For this review, take the finished solid that the model builds, in its own axes (mm). Face numbers are marked on the shaded views. A direction names the side the tool comes from. Coordinates: 2 decimals unless noted, no trailing zeros. Loops run counter-clockwise (first coordinate to the right, second up) from the corner with the lowest first, then second, coordinate; pieces in that order, holes last. Notation, with made-up numbers: M -14.5,31 L 26.5,31 A29 ccw 26.5,59 Z; hole C 11,21 d7. An arc over 180 degrees is marked long. Answer as a JSON object with one key per item and string values. Group by question number.
Item 1: Tool access review of the marked faces 1 and 2: name each direction out of +Z, -Z, +X, -X, +Y, -Y from which nothing blocks a thin tool from reaching the whole face with its end or side.
Item 2: Add section C-C (y = 19). State the section outline as (x, z) points.
Item 3: Add section A-A (y = 7). State the section outline as (x, z) points, then the cut area to 3 significant figures.
Item 4: Add section D-D (x = -3.75). State the section outline as (y, z) points, then the cut area to 3 significant figures.
Item 5: Add section B-B (z = 3). State the section outline as (x, y) points, then the cut area to 3 significant figures.
Item 6: Mouldability with a two-part tool opening along Z and no side actions: class the marked faces 3, 4, 5 and 6 as +Z half, -Z half, draft (parallel to the pull), parting line (faces both ways), or undercut.
Item 7: Wall thickness on L1, parallel to X at y = 1.75, z = 0; L2, parallel to Z at x = 6.5, y = 21.5; L3, parallel to X at y = 0.9, z = 3: over which ranges is each line inside the solid? List them lowest first. Write a range as from..to.
Item 8: Insertion check: pin 1 (5 mm diameter, centred on x = 1.5, z = 0, fed in from +Y); pin 2 (2 mm diameter, centred on y = 20.5, z = -12.5, fed in from +X); pin 3 (2.5 mm diameter, centred on x = 0, z = 3, fed in from +Y); pin 4 (3.5 mm diameter, centred on y = 1.5, z = 1.5, fed in from +X). Each pin has a flat end and moves straight along its axis. Give the tip position at first contact, or say it passes through.
from build123d import *

# Parameters (mm, degrees)
SKETCH_1_W          = 17
SKETCH_1_H          = 23.4
SKETCH_1_R          = 1.6
EXTRUDE_1_DEPTH     = 3
EXTRUDE_3_DEPTH     = 45
SKETCH_3_R          = 1.1
SKETCH_3_R_2        = 5
CUT_EXTRUDE_1_DEPTH = 45
FILLET_1_R          = 2
SKETCH_4_W          = 10
SKETCH_4_H          = 11.187827488
CUT_EXTRUDE_2_DEPTH = 29


with BuildPart() as part:
    # 草图1 → 凸台-拉伸1 (new body)
    with BuildSketch(Plane(origin=(0, 0, 0), x_dir=(1, 0, 0), z_dir=(0, 1, 0))):
        Rectangle(SKETCH_1_W, SKETCH_1_H)
        with Locations(Location((0, 3, 0), (0, 0, 270))):
            Circle(SKETCH_1_R, mode=Mode.SUBTRACT)
        with Locations(Location((-3, 0, 0), (0, 0, 270))):
            Circle(SKETCH_1_R, mode=Mode.SUBTRACT)
        with Locations(Location((0, -3, 0), (0, 0, 90))):
            Circle(SKETCH_1_R, mode=Mode.SUBTRACT)
        with Locations(Location((3, 0, 0), (0, 0, 90))):
            Circle(SKETCH_1_R, mode=Mode.SUBTRACT)
    extrude(amount=EXTRUDE_1_DEPTH)

    # 草图2 → 凸台-拉伸3 (add)
    with BuildSketch(Plane.XZ):
        Polygon((-8.5, 11.7), (-8.5, 13.7), (8.584010661, 13.7), (8.5, 11.7), align=None)
        Polygon((8.584010661, -13.7), (8.5, -11.7), (-8.5, -11.7), (-8.5, -13.7), align=None)
    extrude(amount=-EXTRUDE_3_DEPTH)

    # 草图3 → 切除-拉伸1 (cut)
    with BuildSketch(Plane.XY.offset(13.7)):
        with Locations((-5.707994669, 41)):
            Circle(SKETCH_3_R)
        with Locations((5.792005331, 41)):
            Circle(SKETCH_3_R)
        with Locations((0.042005331, 14)):
            Circle(SKETCH_3_R_2)
        with Locations((-5.707994669, 7)):
            Circle(SKETCH_3_R)
        with Locations((5.792005331, 7)):
            Circle(SKETCH_3_R)
    extrude(amount=-CUT_EXTRUDE_1_DEPTH, mode=Mode.SUBTRACT)

    # 圆角1
    fillet_1_edges = [part.edges().sort_by_distance(p)[0] for p in [
        (-8.5, 45, 12.7),
        (8.542005331, 45, 12.7),
        (-8.5, 45, -12.7),
        (8.542005331, 45, -12.7),
    ]]
    fillet(fillet_1_edges, radius=FILLET_1_R)

    # 草图4 → 切除-拉伸2 (cut)
    with BuildSketch(Plane.XY.offset(13.7)):
        with Locations((0.042005331, 19.593913744)):
            Rectangle(SKETCH_4_W, SKETCH_4_H)
    extrude(amount=-CUT_EXTRUDE_2_DEPTH, mode=Mode.SUBTRACT)


solid = part.part
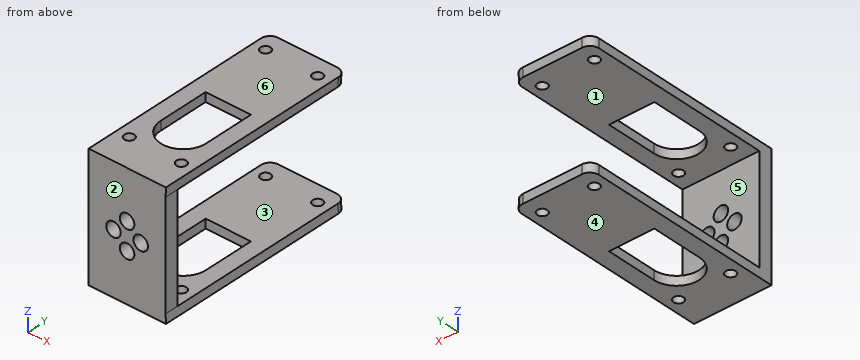
From the geometry:
{
 "1": {"face 1": "+X, -X, +Y", "face 2": "+Z, -Z, +X, -X, -Y"},
 "2": {"outline": "M -8.5,-13.7 L -4.96,-13.7 L -4.96,-11.7 L -8.5,-11.7 Z; M -8.5,11.7 L -4.96,11.7 L -4.96,13.7 L -8.5,13.7 Z; M 5.04,-13.7 L 8.58,-13.7 L 8.5,-11.7 L 5.04,-11.7 Z; M 5.04,11.7 L 8.5,11.7 L 8.58,13.7 L 5.04,13.7 Z"},
 "3": {"outline": "M -8.5,-13.7 L -6.81,-13.7 L -6.81,-11.7 L -8.5,-11.7 Z; M -8.5,11.7 L -6.81,11.7 L -6.81,13.7 L -8.5,13.7 Z; M -4.61,-13.7 L 4.69,-13.7 L 4.69,-11.7 L -4.61,-11.7 Z; M -4.61,11.7 L 4.69,11.7 L 4.69,13.7 L -4.61,13.7 Z; M 6.89,-13.7 L 8.58,-13.7 L 8.5,-11.7 L 6.89,-11.7 Z; M 6.89,11.7 L 8.5,11.7 L 8.58,13.7 L 6.89,13.7 Z", "area": "50.6 mm²"},
 "4": {"outline": "M 0,-13.7 L 10.74,-13.7 L 10.74,-11.7 L 3,-11.7 L 3,-1.41 L 0,-1.41 Z; M 0,1.41 L 3,1.41 L 3,11.7 L 10.74,11.7 L 10.74,13.7 L 0,13.7 Z; M 25.19,-13.7 L 45,-13.7 L 45,-11.7 L 25.19,-11.7 Z; M 25.19,11.7 L 45,11.7 L 45,13.7 L 25.19,13.7 Z", "area": "184 mm²"},
 "5": {"outline": "M -8.5,0 L -1.6,0 L -1.6,3 L -8.5,3 Z; M 1.6,0 L 8.5,0 L 8.5,3 L 1.6,3 Z", "area": "41.4 mm²"},
 "6": {"face 3": "undercut", "face 4": "-Z half", "face 5": "undercut", "face 6": "+Z half"},
 "7": {"L1": "x = -8.5..-4.6, -1.4..1.4, 4.6..8.5", "L2": "z = -13.7..-11.7, 11.7..13.7", "L3": "x = -8.5..-1.6, 1.6..8.5"},
 "8": {"pin 1": "stops at y = 3", "pin 2": "stops at x = 8.58", "pin 3": "passes through", "pin 4": "stops at x = 8.5"}
}
